The model under review builds one solid part; all positions refer to its coordinate system, in mm. A direction names the side the tool comes from. Round coordinates to 2 decimals unless told otherwise and drop trailing zeros. Order: outer loops, then holes, each group sorted by start corner. A loop starts at its lowest first (then second) coordinate and runs counter-clockwise, first axis right, second up. Notation, with made-up numbers: (-7.5, 69.25) -> (21.5, 69.25) arc R13 cw to (21.5, 88.25) -> close; hole circle Ø7 at (49, 61). An arc over 180 degrees is marked (long way). Use a Markdown table: item, result. Add a question column.
```python
from build123d import *
from build123d.topology import SkipClean

# Parameters (mm, degrees)
SKETCH1_R                = 90
BOSS_EXTRUDE1_DEPTH      = 50
CUT_EXTRUDE1_DEPTH       = 50
SKETCH4_R                = 40
CUT_EXTRUDE2_DEPTH       = 137.546695512
SKETCH5_R                = 40
SKETCH5_R_2              = 34
BOSS_EXTRUDE2_DEPTH      = 50
BOSS_EXTRUDE3_DEPTH      = 15
BOSS_EXTRUDE3_DEPTH_BACK = 15
SKETCH9_R                = 34
SKETCH9_R_2              = 30
SKETCH10_R               = 40
SKETCH10_R_2             = 30
BOSS_EXTRUDE4_DEPTH      = 10.5
SKETCH11_R               = 90
SKETCH11_R_2             = 87
BOSS_EXTRUDE5_DEPTH      = 50
SKETCH12_R               = 87
SKETCH12_R_2             = 40
CUT_EXTRUDE3_DEPTH       = 4
SKETCH13_R               = 87
CUT_EXTRUDE4_DEPTH       = 4


with BuildPart() as part:
    # Sketch1 → Boss-Extrude1 (new body)
    with BuildSketch(Plane(origin=(0, 0, 0), x_dir=(1, 0, 0), z_dir=(0, 1, 0))):
        with Locations(Location((0, 0, 0), (0, 0, 270))):
            Circle(SKETCH1_R)
    extrude(amount=BOSS_EXTRUDE1_DEPTH)

    # Sketch2 → Cut-Extrude1 (cut)
    with BuildSketch(Plane.XZ):
        with BuildLine():
            Line((-2, 9.409260219), (-2, 89.977775034))
            ThreePointArc((-2, 89.977775034), (-18.712052174, 88.033284066), (-34.770167253, 83.012260957))
            Line((-34.770167253, 83.012260957), (-2, 9.409260219))
        make_face()
        with BuildLine():
            ThreePointArc((34.770167253, 83.012260957), (18.712052174, 88.033284066), (2, 89.977775034))
            Line((2, 89.977775034), (2, 9.409260219))
            Line((2, 9.409260219), (34.770167253, 83.012260957))
        make_face()
        with BuildLine():
            Line((-5.654181831, 7.782313647), (-38.424349084, 81.385314385))
            ThreePointArc((-38.424349084, 81.385314385), (-52.900672706, 72.811529494), (-65.528256711, 61.693172818))
            Line((-65.528256711, 61.693172818), (-5.654181831, 7.782313647))
        make_face()
        with BuildLine():
            ThreePointArc((65.528256711, 61.693172818), (52.900672706, 72.811529494), (38.424349084, 81.385314385))
            Line((38.424349084, 81.385314385), (5.654181831, 7.782313647))
            Line((5.654181831, 7.782313647), (65.528256711, 61.693172818))
        make_face()
        with BuildLine():
            Line((-8.330704256, 4.809734345), (-68.204779137, 58.720593516))
            ThreePointArc((-68.204779137, 58.720593516), (-77.942286341, 45), (-84.955915279, 29.706774634))
            Line((-84.955915279, 29.706774634), (-8.330704256, 4.809734345))
        make_face()
        with BuildLine():
            ThreePointArc((84.955915279, 29.706774634), (77.942286341, 45), (68.204779137, 58.720593516))
            Line((68.204779137, 58.720593516), (8.330704256, 4.809734345))
            Line((8.330704256, 4.809734345), (84.955915279, 29.706774634))
        make_face()
        with BuildLine():
            Line((-9.566772234, 1.00550828), (-86.191983256, 25.902548569))
            ThreePointArc((-86.191983256, 25.902548569), (-89.506970583, 9.407561694), (-89.693924294, -7.416194762))
            Line((-89.693924294, -7.416194762), (-9.566772234, 1.00550828))
        make_face()
        with BuildLine():
            ThreePointArc((89.693924294, -7.416194762), (89.506970583, 9.407561694), (86.191983256, 25.902548569))
            Line((86.191983256, 25.902548569), (9.566772234, 1.00550828))
            Line((9.566772234, 1.00550828), (89.693924294, -7.416194762))
        make_face()
        with BuildLine():
            Line((-9.14865838, -2.972579302), (-89.275810441, -11.394282343))
            ThreePointArc((-89.275810441, -11.394282343), (-85.595086467, -27.811529494), (-78.923038955, -43.256836709))
            Line((-78.923038955, -43.256836709), (-9.14865838, -2.972579302))
        make_face()
        with BuildLine():
            Line((89.275810441, -11.394282343), (9.14865838, -2.972579302))
            Line((9.14865838, -2.972579302), (78.923038955, -43.256836709))
            ThreePointArc((78.923038955, -43.256836709), (85.595086467, -27.811529494), (89.275810441, -11.394282343))
        make_face()
        with BuildLine():
            Line((-7.14865838, -6.436680917), (-76.923038955, -46.720938324))
            ThreePointArc((-76.923038955, -46.720938324), (-66.883034293, -60.221754572), (-54.505643188, -71.617978614))
            Line((-54.505643188, -71.617978614), (-7.14865838, -6.436680917))
        make_face()
        with BuildLine():
            Line((76.923038955, -46.720938324), (7.14865838, -6.436680917))
            Line((7.14865838, -6.436680917), (54.505643188, -71.617978614))
            ThreePointArc((54.505643188, -71.617978614), (66.883034293, -60.221754572), (76.923038955, -46.720938324))
        make_face()
        with BuildLine():
            Line((-3.912590403, -8.787821926), (-51.26957521, -73.969119623))
            ThreePointArc((-51.26957521, -73.969119623), (-36.606297877, -82.219091188), (-20.663726545, -87.595721387))
            Line((-20.663726545, -87.595721387), (-3.912590403, -8.787821926))
        make_face()
        with BuildLine():
            Line((51.26957521, -73.969119623), (3.912590403, -8.787821926))
            Line((3.912590403, -8.787821926), (20.663726545, -87.595721387))
            ThreePointArc((20.663726545, -87.595721387), (36.606297877, -82.219091188), (51.26957521, -73.969119623))
        make_face()
        with BuildLine():
            Line((0, -9.619468689), (-16.751136142, -88.42736815))
            ThreePointArc((-16.751136142, -88.42736815), (0, -90), (16.751136142, -88.42736815))
            Line((16.751136142, -88.42736815), (0, -9.619468689))
        make_face()
    extrude(amount=-CUT_EXTRUDE1_DEPTH, mode=Mode.SUBTRACT)

    # Sketch4 → Cut-Extrude2 (cut, through all)
    with BuildSketch(Plane(origin=(0, 50, 0), x_dir=(1, 0, 0), z_dir=(0, 1, 0))):
        Circle(SKETCH4_R)
    extrude(amount=-CUT_EXTRUDE2_DEPTH, mode=Mode.SUBTRACT)


with BuildPart() as cut_extrude2_piece_1:
    # of the separate pieces the step leaves, piece 1, a body of its own (cut_extrude2_pieces)
    add(part.part.solids().sort_by_distance((-84.955915279, 0, 29.706774634))[0])


with BuildPart() as cut_extrude2_piece_2:
    # of the separate pieces the step leaves, piece 2, a body of its own (cut_extrude2_pieces)
    add(part.part.solids().sort_by_distance((-65.528256711, 0, 61.693172818))[0])


with BuildPart() as cut_extrude2_piece_3:
    # of the separate pieces the step leaves, piece 3, a body of its own (cut_extrude2_pieces)
    add(part.part.solids().sort_by_distance((10.262360744, 0, -38.661142662))[0])


with BuildPart() as cut_extrude2_piece_4:
    # of the separate pieces the step leaves, piece 4, a body of its own (cut_extrude2_pieces)
    add(part.part.solids().sort_by_distance((14.422025249, 0, 37.309585735))[0])


with BuildPart() as cut_extrude2_piece_5:
    # of the separate pieces the step leaves, piece 5, a body of its own (cut_extrude2_pieces)
    add(part.part.solids().sort_by_distance((-2, 0, 89.977775034))[0])


with BuildPart() as cut_extrude2_piece_6:
    # of the separate pieces the step leaves, piece 6, a body of its own (cut_extrude2_pieces)
    add(part.part.solids().sort_by_distance((39.940175529, 0, -2.186865046))[0])


with BuildPart() as cut_extrude2_piece_7:
    # of the separate pieces the step leaves, piece 7, a body of its own (cut_extrude2_pieces)
    add(part.part.solids().sort_by_distance((25.100036427, 0, -31.144633107))[0])


with BuildPart() as cut_extrude2_piece_8:
    # of the separate pieces the step leaves, piece 8, a body of its own (cut_extrude2_pieces)
    add(part.part.solids().sort_by_distance((-34.770167253, 0, 83.012260957))[0])


with BuildPart() as cut_extrude2_piece_9:
    # of the separate pieces the step leaves, piece 9, a body of its own (cut_extrude2_pieces)
    add(part.part.solids().sort_by_distance((28.350351313, 0, 28.218036438))[0])


with BuildPart() as cut_extrude2_piece_10:
    # of the separate pieces the step leaves, piece 10, a body of its own (cut_extrude2_pieces)
    add(part.part.solids().sort_by_distance((-20.663726545, 0, -87.595721387))[0])


with BuildPart() as cut_extrude2_piece_11:
    # of the separate pieces the step leaves, piece 11, a body of its own (cut_extrude2_pieces)
    add(part.part.solids().sort_by_distance((-54.505643188, 0, -71.617978614))[0])


with BuildPart() as cut_extrude2_piece_12:
    # of the separate pieces the step leaves, piece 12, a body of its own (cut_extrude2_pieces)
    add(part.part.solids().sort_by_distance((37.37664408, 0, 14.247332289))[0])


with BuildPart() as cut_extrude2_piece_13:
    # of the separate pieces the step leaves, piece 13, a body of its own (cut_extrude2_pieces)
    add(part.part.solids().sort_by_distance((35.597687784, 0, -18.242933548))[0])


with BuildPart() as cut_extrude2_piece_14:
    # of the separate pieces the step leaves, piece 14, a body of its own (cut_extrude2_pieces)
    add(part.part.solids().sort_by_distance((-89.693924294, 0, -7.416194762))[0])


with BuildPart() as cut_extrude2_piece_15:
    # of the separate pieces the step leaves, piece 15, a body of its own (cut_extrude2_pieces)
    add(part.part.solids().sort_by_distance((-78.923038955, 0, -43.256836709))[0])


with BuildPart() as body_16:
    # Sketch5 → Boss-Extrude2 (new body)
    with BuildSketch(Plane(origin=(0, 50, 0), x_dir=(1, 0, 0), z_dir=(0, 1, 0))):
        with Locations(Location((0, 0, 0), (0, 0, 270))):
            Circle(SKETCH5_R)
        with Locations(Location((0, 0, 0), (0, 0, 270))):
            Circle(SKETCH5_R_2, mode=Mode.SUBTRACT)
    extrude(amount=-BOSS_EXTRUDE2_DEPTH)



with BuildPart() as body_17:
    # Sketch9 → Boss-Extrude3 (new, two sides: drawn at the far end of the back side and taken through both)
    with BuildSketch(Plane(origin=(0, 50, 0), x_dir=(1, 0, 0), z_dir=(0, 1, 0)).offset(-BOSS_EXTRUDE3_DEPTH_BACK)):
        with Locations(Location((0, 0, 0), (0, 0, 270))):
            Circle(SKETCH9_R)
        with Locations(Location((0, 0, 0), (0, 0, 270))):
            Circle(SKETCH9_R_2, mode=Mode.SUBTRACT)
    extrude(amount=BOSS_EXTRUDE3_DEPTH + BOSS_EXTRUDE3_DEPTH_BACK)

    # Sketch10 → Boss-Extrude4 (add)
    with BuildSketch(Plane(origin=(0, 65, 0), x_dir=(1, 0, 0), z_dir=(0, 1, 0))):
        with Locations(Location((0, 0, 0), (0, 0, 270))):
            Circle(SKETCH10_R)
        with Locations(Location((0, 0, 0), (0, 0, 270))):
            Circle(SKETCH10_R_2, mode=Mode.SUBTRACT)
    extrude(amount=BOSS_EXTRUDE4_DEPTH)


with BuildPart() as body_16_1:
    add(body_16.part)

    add(body_17.part)  # Boss-Extrude5 merges body 17

    add(cut_extrude2_piece_3.part)  # Boss-Extrude5 merges Cut-Extrude2 piece 3

    add(cut_extrude2_piece_7.part)  # Boss-Extrude5 merges Cut-Extrude2 piece 7

    add(cut_extrude2_piece_14.part)  # Boss-Extrude5 merges Cut-Extrude2 piece 14

    add(cut_extrude2_piece_15.part)  # Boss-Extrude5 merges Cut-Extrude2 piece 15

    add(cut_extrude2_piece_11.part)  # Boss-Extrude5 merges Cut-Extrude2 piece 11

    add(cut_extrude2_piece_5.part)  # Boss-Extrude5 merges Cut-Extrude2 piece 5

    add(cut_extrude2_piece_1.part)  # Boss-Extrude5 merges Cut-Extrude2 piece 1

    add(cut_extrude2_piece_8.part)  # Boss-Extrude5 merges Cut-Extrude2 piece 8

    add(cut_extrude2_piece_2.part)  # Boss-Extrude5 merges Cut-Extrude2 piece 2

    add(cut_extrude2_piece_13.part)  # Boss-Extrude5 merges Cut-Extrude2 piece 13

    add(cut_extrude2_piece_6.part)  # Boss-Extrude5 merges Cut-Extrude2 piece 6

    add(cut_extrude2_piece_4.part)  # Boss-Extrude5 merges Cut-Extrude2 piece 4

    add(cut_extrude2_piece_12.part)  # Boss-Extrude5 merges Cut-Extrude2 piece 12

    add(cut_extrude2_piece_9.part)  # Boss-Extrude5 merges Cut-Extrude2 piece 9

    add(cut_extrude2_piece_10.part)  # Boss-Extrude5 merges Cut-Extrude2 piece 10
    # Sketch11 → Boss-Extrude5 (add)
    with BuildSketch(Plane.XZ):
        with Locations(Location((0, 0, 0), (0, 0, 90))):
            Circle(SKETCH11_R)
        Circle(SKETCH11_R_2, mode=Mode.SUBTRACT)
    extrude(amount=-BOSS_EXTRUDE5_DEPTH)

    # Sketch12 → Cut-Extrude3 (cut)
    with SkipClean():  # the faces are left unmerged after this step: merging them gives an invalid solid
        with BuildSketch(Plane(origin=(0, 50, 0), x_dir=(1, 0, 0), z_dir=(0, 1, 0))):
            with Locations(Location((0, 0, 0), (0, 0, 100.682739604))):
                Circle(SKETCH12_R)
            with Locations(Location((0, 0, 0), (0, 0, 270))):
                Circle(SKETCH12_R_2, mode=Mode.SUBTRACT)
        extrude(amount=-CUT_EXTRUDE3_DEPTH, mode=Mode.SUBTRACT)
    add(body_16_1.part.scale(1), mode=Mode.REPLACE)  # the faces are merged on a copy

    # Sketch13 → Cut-Extrude4 (cut)
    with SkipClean():  # the faces are left unmerged after this step: merging them gives an invalid solid
        with BuildSketch(Plane.XZ):
            with Locations(Location((0, 0, 0), (0, 0, 270))):
                Circle(SKETCH13_R)
        extrude(amount=-CUT_EXTRUDE4_DEPTH, mode=Mode.SUBTRACT)


solid = body_16_1.part
```
Q1. Add section B-B (y = 53). Write out the cut boundary in (x, z).
Q2. Add section D-D (y = 67.5). Write out the cut boundary in (x, z), then the cut area to 3 significant figures.
Q3. Wall thickness on line 1 (X direction, y = 48, z = 0); line 2 (X direction, y = 25, z = 0); line 3 (Z direction, x = -67, y = 34.5): over which ranges is each line inside the solid? List them lowest first. Write a range as [from, to].
Q4. Add section C-C (z = 50). Write out the cut boundary in (x, y), then the cut area to 3 significant figures.
Q5. Machinability: for faces 3 (the cylindrical face through (-39.05, 70.18, -8.67)), 4 (the flat face through (45.58, 24.71, 43.73)), which of the approach directions +Z, -Z, +X, -X, +Y, -Y give a long, thin tool a straight path to every point of the face, cutting with its end or side? Answer none if there is none.
Q6. Mouldability with a two-part tool opening along Z and no side actions: class faces 1 (the cylindrical face through (-56.337, 24.65, -70.186)), 2 (the flat face through (48.745, 24.706, 41.199)) as pulls with the +Z half, pulls with the -Z half, needs draft (parallel to the pull), parting line crosses it, or undercut.
Q7. Add section A-A (z = 0). Write out the cut boundary in (x, y), then the cut area to 3 significant figures.
Q8. Insertion check: pin 1 (7 mm diameter, centred on x = 56, z = -5.5, fed in from +Y); pin 2 (12 mm diameter, centred on x = -30, y = 29, fed in from -Z); pin 3 (1 mm diameter, centred on x = 51.5, z = 48, fed in from -Y). Each pin has a flat end and moves straight along its axis. Give the tip position at first contact, or say it passes through.
Report:
| question | item | result |
|---|---|---|
| 1 | outline | circle Ø68 at (0, 0); hole circle Ø60 at (0, 0) |
| 2 | outline | circle Ø80 at (0, 0); hole circle Ø60 at (0, 0) |
| 2 | area | 2,200 mm² |
| 3 | line 1 | x = [-90, -87], [-40, -30], [30, 40], [87, 90] |
| 3 | line 2 | x = [-90, -87], [-40, -34], [34, 40], [87, 90] |
| 3 | line 3 | z = [-60.09, -55.5], [-40.99, -36.37], [-9.05, -5.03], [19.67, 23.87], [55.5, 60.09] |
| 4 | outline | (-74.83, 0) -> (-71.2, 0) -> (-71.2, 50) -> (-74.83, 50) -> close; (-58.52, 4) -> (-52.54, 4) -> (-52.54, 46) -> (-58.52, 46) -> close; (-24.45, 4) -> (-20.07, 4) -> (-20.07, 46) -> (-24.45, 46) -> close; (-2, 4) -> (2, 4) -> (2, 46) -> (-2, 46) -> close; (20.07, 4) -> (24.45, 4) -> (24.45, 46) -> (20.07, 46) -> close; (52.54, 4) -> (58.52, 4) -> (58.52, 46) -> (52.54, 46) -> close; (71.2, 0) -> (74.83, 0) -> (74.83, 50) -> (71.2, 50) -> close |
| 4 | area | 1,400 mm² |
| 5 | face 3 | +Y |
| 5 | face 4 | +Y, -Y |
| 6 | face 1 | parting line crosses it |
| 6 | face 2 | undercut |
| 7 | outline | (-90, 0) -> (-87, 0) -> (-87, 50) -> (-90, 50) -> close; (-40, 4) -> (-34, 4) -> (-34, 35) -> (-30, 35) -> (-30, 75.5) -> (-40, 75.5) -> (-40, 65) -> (-34, 65) -> (-34, 50) -> (-40, 50) -> close; (30, 35) -> (34, 35) -> (34, 4) -> (40, 4) -> (40, 50) -> (34, 50) -> (34, 65) -> (40, 65) -> (40, 75.5) -> (30, 75.5) -> close; (87, 0) -> (90, 0) -> (90, 50) -> (87, 50) -> close |
| 7 | area | 1,300 mm² |
| 8 | pin 1 | stops at y = 46 |
| 8 | pin 2 | stops at z = -86.74 |
| 8 | pin 3 | stops at y = 4 |
